Autodesk Inventor part; units mm, degrees
ref_plane "YZ Plane" through (0, 0, 0) normal (1, 0, 0) x (0, 1, 0)
ref_plane "XZ Plane" through (0, 0, 0) normal (0, 1, 0) x (-1, 0, 0)
ref_plane "XY Plane" through (0, 0, 0) normal (0, 0, 1) x (1, 0, 0)
sketch "Esboço1" plane through (0, 0, 0) normal (0, 0, 1) x (1, 0, 0)
  line L0 (7.5, 7.5) -> (-7.5, 7.5) construction
  line L1 (-7.5, 3.1) -> (-7.5, -3.1) construction
  line L2 (-7.5, 7.5) -> (-7.5, 3.1) construction
  line L3 (-7.5, 3.1) -> (-5.5, 3.1) construction
  line L4 (-5.5, 3.1) -> (-5.5, 6.2) construction
  line L5 (-5.5, 6.2) -> (-1.5, 3.1) construction
  line L6 (-1.5, 3.1) -> (-1.5, 0) construction
  line L7 (-1.5, 0) -> (0, 0)
  line L8 (0, 0) -> (0, 7.5)
  arc A0 (-7, 7.5) -> (-7.5, 7) centre (-7, 7) ccw
  line L9 (-7.5, 3.1) -> (-7, 3.1) construction
  line L10 (-7, 3.1) -> (-7, 3.6)
  line L11 (-7, 3.6) -> (-7.5, 3.6)
  line L12 (-7.5, 3.6) -> (-7.5, 3.1) construction
  line L13 (-7.5, 7) -> (-7.5, 3.6)
  line L14 (-7, 7.5) -> (0, 7.5)
  line L15 (-7, 3.1) -> (-5.5, 3.1)
  arc A1 (-5.1775, 5.9501) -> (-5.5, 5.792) centre (-5.3, 5.792) ccw
  line L16 (-5.5, 3.1) -> (-5.5, 5.792)
  arc A2 (-1.5, 2.8549) -> (-1.6937, 3.2501) centre (-2, 2.8549) ccw
  line L17 (-5.1775, 5.9501) -> (-1.6937, 3.2501)
  line L18 (-1.5, 2.8549) -> (-1.5, 0)
  point P0 (-7.5, 0)
  dimension "d0" = 15
  dimension "d1" = 6.2
  dimension "d2" = 7.5
  dimension "d4" = 2
  dimension "d5" = 6
  dimension "d7" = 3.1
  dimension "d10" = 0.5
  dimension "d11" = 0.5
  dimension "d12" = 0.2
  dimension "d13" = 0.5
extrude "Extrusão1" add sketch "Esboço1" along normal mid plane 2000
mirror "Espelhar1" about plane through (0, 0, 0) normal (1, 0, 0) of "Extrusão1"
mirror "Espelhar2" about plane through (0, 0, 0) normal (0, 1, 0) of "Extrusão1", "Espelhar1"
equation "\"d2\" = 0.5 * d0"
properties part number "15×15 2 slots profile_AST01501502" material "Alumínio 6061"
Part model, mm, in its own coordinate system. Coordinates: 2 decimals unless noted, no trailing zeros. Loops run counter-clockwise (first coordinate to the right, second up) from the corner with the lowest first, then second, coordinate; pieces in that order, holes last. Notation, with made-up numbers: M -21,74 L 26,74 A15 cw 26,82 Z; hole C 19,22.25 d10. An arc over 180 degrees is marked long. Use a Markdown table: item, result. Add a question column.
Q1. Pin check, flat tips, straight feed: P1, Ø0.6, axis at y = -3, z = 98.5, coming from the -X side; P2, Ø1, axis at y = -2.5, z = -163, coming from the +X side. Stop position of each tip, or through.
Q2. Probe L1, parallel to X at y = -5.75, z = -661.5; L2, parallel to X at y = 5, z = -534; L3, parallel to Y at x = -2, z = 752.5. List the from-to ranges inside material, lowest first.
Q3. Cut at A-A (y = -0.5). Write the cut outline in (x, z).
Worked out:
| question | item | result |
|---|---|---|
| 1 | P1 | stops at x = -7 |
| 1 | P2 | stops at x = 1.52 |
| 2 | L1 | x = -7.5 to -5.5, -4.92 to 4.92, 5.5 to 7.5 |
| 2 | L2 | x = -7.5 to -5.5, -3.95 to 3.95, 5.5 to 7.5 |
| 2 | L3 | y = -7.5 to -3.49, 3.49 to 7.5 |
| 3 | outline | M -1.5,-1000 L 1.5,-1000 L 1.5,1000 L -1.5,1000 Z |
